Read the model definition and answer for the solid it produces. Units are mm, in the model's axes. Face numbers are marked on the shaded views. A direction names the side the tool comes from. Coordinates: 2 decimals unless noted, no trailing zeros. Order: outer loops, then holes, each group sorted by start corner. A loop starts at its lowest first (then second) coordinate and runs counter-clockwise, first axis right, second up. Notation, with made-up numbers: M 13.25,8.5 L 62.25,8.5 A18 cw 62.25,40.5 Z; hole C 24.25,-24.5 d3. An arc over 180 degrees is marked long. Use a Markdown table: item, result. Add a question column.
1) Each of these flat-tipped pins is pushed along its axis until it touches: pin 1 Ø12.5 at (x, y) = (-54, 60) entering from +Z; pin 2 Ø10 at (x, z) = (15.5, 10) entering from +Y; pin 3 Ø8 at (x, z) = (7, 3) entering from +Y; pin 4 Ø2 at (x, z) = (38, 13.5) entering from +Y. Where does it stop, or does it pass through?
2) Find the intervals of material crossed by probe 1 along Y at (x, z) = (-54, 16.25); probe 2 along Y at (x, z) = (0, 14); probe 3 along X at (y, z) = (26.5, 9.25), in increasing order. Write a range as [from, to].
3) Find section D-D on y = -60. Write down the section's boundary in (x, z), plus the area to 3 significant figures.
4) For the marked faces 4 and 5, determine the directions among +Z, -Z, +X, -X, +Y, -Y from which every point of the face is accessible in a straight line to the end or side of a thin tool.
5) Find section C-C on x = -20. Write down the section's boundary in (y, z).
6) The mould has two halves that part along X. Classify the marked faces 1, 2 and 3: released by +X, released by -X, zero draft, split by the parting line, or undercut.
7) Find section B-B on x = 0. Write down the section's boundary in (y, z).
8) Find section A-A on y = 23.5. Write down the section's boundary in (x, z).
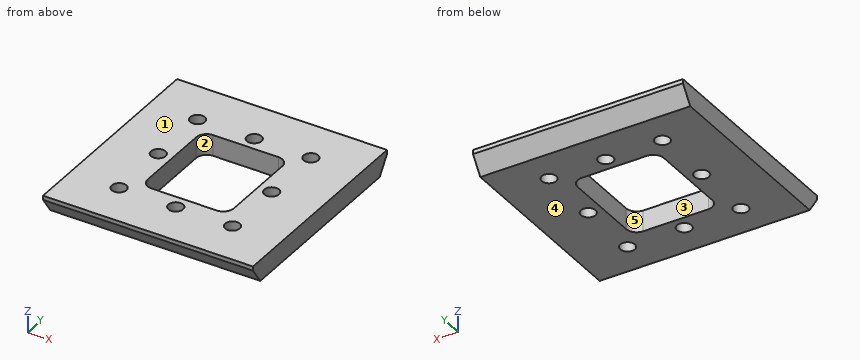
from build123d import *

# Parameters (mm, degrees)
SKETCH_1_W          = 200
SKETCH_1_H          = 205
EXTRUDE_1_DEPTH     = 20
SKETCH_2_R          = 7
CUT_EXTRUDE_1_DEPTH = 145.589937409
CUT_EXTRUDE_2_DEPTH = 226.624134347


with BuildPart() as part:
    # 草图1 → 凸台-拉伸1 (new body)
    with BuildSketch(Plane.XY):
        Rectangle(SKETCH_1_W, SKETCH_1_H)
    extrude(amount=EXTRUDE_1_DEPTH)

    # 草图2 → 切除-拉伸1 (cut, through all)
    with BuildSketch(Plane.XY.offset(20)):
        with Locations((-54, 60)):
            Circle(SKETCH_2_R)
        with Locations((0, 60)):
            Circle(SKETCH_2_R)
        with Locations((-54, 0)):
            Circle(SKETCH_2_R)
        with Locations(Location((54, 0, 0), (0, 0, 180))):
            Circle(SKETCH_2_R)
        with Locations(Location((54, 60, 0), (0, 0, 180))):
            Circle(SKETCH_2_R)
        with Locations(Location((-54, -60, 0), (0, 0, 180))):
            Circle(SKETCH_2_R)
        with Locations(Location((0, -60, 0), (0, 0, 180))):
            Circle(SKETCH_2_R)
        with Locations((54, -60)):
            Circle(SKETCH_2_R)
        with BuildLine():
            Line((-31, 47), (31, 47))
            ThreePointArc((31, 47), (38.071067812, 44.071067812), (41, 37))
            Line((41, 37), (41, -37))
            ThreePointArc((41, -37), (38.071067812, -44.071067812), (31, -47))
            Line((31, -47), (-31, -47))
            ThreePointArc((-31, -47), (-38.071067812, -44.071067812), (-41, -37))
            Line((-41, -37), (-41, 37))
            ThreePointArc((-41, 37), (-38.071067812, 44.071067812), (-31, 47))
        make_face()
    extrude(amount=-CUT_EXTRUDE_1_DEPTH, mode=Mode.SUBTRACT)

    # 草图3 → 切除-拉伸2 (cut, through all)
    with BuildSketch(Plane.ZY.offset(100)):
        Polygon((0, 102.5), (0, 91.296679389), (16, 102.5), align=None)
        Polygon((0, -102.5), (16, -102.5), (0, -91.296679389), align=None)
    extrude(amount=-CUT_EXTRUDE_2_DEPTH, mode=Mode.SUBTRACT)


solid = part.part
Check result:
| question | item | result |
|---|---|---|
| 1 | pin 1 | passes through |
| 1 | pin 2 | stops at y = 101.8 |
| 1 | pin 3 | stops at y = 96.2 |
| 1 | pin 4 | stops at y = 101.45 |
| 2 | probe 1 | y = [-102.5, -67], [-53, -7], [7, 53], [67, 102.5] |
| 2 | probe 2 | y = [-101.1, -67], [-53, -47], [47, 53], [67, 101.1] |
| 2 | probe 3 | x = [-100, -41], [41, 100] |
| 3 | outline | M -100,0 L -61,0 L -61,20 L -100,20 Z; M -47,0 L -7,0 L -7,20 L -47,20 Z; M 7,0 L 47,0 L 47,20 L 7,20 Z; M 61,0 L 100,0 L 100,20 L 61,20 Z |
| 3 | area | 3,160 mm2 |
| 4 | face 4 | -Z, +X, -X, +Y, -Y |
| 4 | face 5 | +Z, -Z |
| 5 | outline | M -102.5,16 L -91.3,0 L -47,0 L -47,20 L -102.5,20 Z; M 47,0 L 91.3,0 L 102.5,16 L 102.5,20 L 47,20 Z |
| 6 | face 1 | zero draft |
| 6 | face 2 | undercut |
| 6 | face 3 | undercut |
| 7 | outline | M -102.5,16 L -91.3,0 L -67,0 L -67,20 L -102.5,20 Z; M -53,0 L -47,0 L -47,20 L -53,20 Z; M 47,0 L 53,0 L 53,20 L 47,20 Z; M 67,0 L 91.3,0 L 102.5,16 L 102.5,20 L 67,20 Z |
| 8 | outline | M -100,0 L -41,0 L -41,20 L -100,20 Z; M 41,0 L 100,0 L 100,20 L 41,20 Z |
